Design review of the part built by this model. Coordinates are the model's own, in mm. A direction names the side the tool comes from. Give positions to 0.01 mm unless a question says otherwise; leave off trailing zeros. Loops run counter-clockwise (first coordinate to the right, second up) from the corner with the lowest first, then second, coordinate; pieces in that order, holes last.
from build123d import *

# Parameters (mm, degrees)
SKETCH_1_W          = 12
SKETCH_1_H          = 12
EXTRUDE_1_DEPTH     = 7
SKETCH_2_W          = 24
SKETCH_2_H          = 35
EXTRUDE_2_DEPTH     = 2
SKETCH_3_W          = 9
SKETCH_3_H          = 7
EXTRUDE_3_DEPTH     = 2
SKETCH_4_R          = 2
CUT_EXTRUDE_1_DEPTH = 2


with BuildPart() as part:
    # 스케치1 → 보스-돌출1 (new body)
    with BuildSketch(Plane.XY):
        Rectangle(SKETCH_1_W, SKETCH_1_H)
    extrude(amount=EXTRUDE_1_DEPTH)

    # 스케치2 → 보스-돌출2 (add)
    with BuildSketch(Plane(origin=(0, 0, 0), x_dir=(-1, 0, 0), z_dir=(0, 0, -1))):
        with Locations((0, -9)):
            Rectangle(SKETCH_2_W, SKETCH_2_H)
    extrude(amount=EXTRUDE_2_DEPTH)

    # 스케치3 → 보스-돌출3 (add)
    with BuildSketch(Plane.XY):
        with Locations((0, -23)):
            Rectangle(SKETCH_3_W, SKETCH_3_H)
    extrude(amount=EXTRUDE_3_DEPTH)

    # 스케치4 → 컷-돌출1 (cut)
    with BuildSketch(Plane.XY.offset(7)):
        Circle(SKETCH_4_R)
    extrude(amount=-CUT_EXTRUDE_1_DEPTH, mode=Mode.SUBTRACT)


solid = part.part
Q1. Take a section at B-B (y = 0). Give the boundary of the cut face in (x, z), plus the area to 3 significant figures.
Results:
outline: (-12, -2) - (12, -2) - (12, 0) - (6, 0) - (6, 7) - (2, 7) - (2, 5) - (-2, 5) - (-2, 7) - (-6, 7) - (-6, 0) - (-12, 0) - close
area: 124 mm2
Q2. Tool access review of faces 1 (the face through (0, -23, 2)), 2 (the face through (0, 6, 3)), 3 (the face through (6, 0, 3)), 4 (the face through (-4.5, -23, 1)), 5 (the face through (0, -19.5, 1)): name each direction out of +Z, -Z, +X, -X, +Y, -Y from which nothing blocks a thin tool from reaching the whole face with its end or side.
Results:
face 1: +Z, +X, -X, -Y
face 2: +Z, +X, -X, +Y
face 3: +Z, +X, +Y, -Y
face 4: +Z, -X, -Y
face 5: +Z, +X, -X
Q3. Insertion check: pin 1 (2 mm diameter, centred on y = 2.5, z = 2.5, fed in from -X); pin 2 (2 mm diameter, centred on y = -22.5, z = 1.5, fed in from +X); pin 3 (2 mm diameter, centred on x = -1, z = 3, fed in from +Y). Each pin has a flat end and moves straight along its axis. Give the tip position at first contact, or say it passes through.
Results:
pin 1: stops at x = -6
pin 2: stops at x = 4.5
pin 3: stops at y = 6
Q4. Take a section at A-A (x = 3.5). Give the boundary of the cut face in (y, z).
Results:
outline: (-26.5, -2) - (8.5, -2) - (8.5, 0) - (6, 0) - (6, 7) - (-6, 7) - (-6, 0) - (-19.5, 0) - (-19.5, 2) - (-26.5, 2) - close
Q5. Wall thickness on line 1 (Y direction, x = 0, z = 6.25); line 2 (Z direction, x = -8, y = -24); line 3 (Z direction, x = 1, y = -25): over which ranges is each line inside the solid? List them lowest first.
Results:
line 1: y = -6 to -2, 2 to 6
line 2: z = -2 to 0
line 3: z = -2 to 2
Q6. Take a section at D-D (x = 0). Give the boundary of the cut face in (y, z).
Results:
outline: (-26.5, -2) - (8.5, -2) - (8.5, 0) - (6, 0) - (6, 7) - (2, 7) - (2, 5) - (-2, 5) - (-2, 7) - (-6, 7) - (-6, 0) - (-19.5, 0) - (-19.5, 2) - (-26.5, 2) - close
Q7. Take a section at C-C (z = 4.25). Give the boundary of the cut face in (x, y), plus the area to 3 significant figures.
Results:
outline: (-6, -6) - (6, -6) - (6, 6) - (-6, 6) - close
area: 144 mm2
Q8. Draft analysis for pull direction Y (two halves, no side actions). For faces 6 (the face through (0, 0, 5)), 7 (the face through (0, 8.5, -1)), 8 (the face through (4.5, -23, 1)), state which applies: pulls with the +Y half, pulls with the -Y half, needs draft (parallel to the pull), parting line crosses it, or undercut.
Results:
face 6: undercut
face 7: pulls with the +Y half
face 8: needs draft
